Source: CAD feature listing. Evaluate the final solid. Frame: model axes, mm. Give positions to 0.01 mm unless a question says otherwise; leave off trailing zeros. Write each loop counter-clockwise with the first axis right and the second up, starting at its lowest first coordinate (ties: lowest second). Pieces come first, ordered by that corner, then holes. Notation, with made-up numbers: (71, 56) -> (120, 56) arc R28 cw to (120, 84) -> close; hole circle Ø9 at (-9.75, 31.25). An arc over 180 degrees is marked (long way). Answer as a JSON object with one key per item and string values. Group by question number.
Item 1: Section query B-B on x = 134.5. Return the cut outline in (y, z).
Item 2: Section query A-A on x = 260. Return the cut outline in (y, z).
Item 3: Section query C-C on y = 0.95. Give the number of separate pieces and of enclosed holes in the cut face, plus the area to 3 significant figures.
Item 4: First-contact query: pin 1 Ø1.5 at (y, z) = (1, -13) entering from +X; pin 2 Ø1.5 at (x, y) = (202.5, 1.5) entering from -Z; pin 3 Ø1.5 at (y, z) = (2, -16) entering from -X. Flat tips, straight axial feed; report the tip coordinate or a pass-through.
Item 5: Ray query, probe 1 along X at (y, z) = (2.1, -16); probe 2 along X at (y, z) = (2.75, -6.75); probe 3 along Z at (x, y) = (35.5, 1). Return the intervals inside material, ascending. Write a range as from..to.
Item 6: Section query D-D on x = 51. Return the cut outline in (y, z).
from build123d import *

# Parameters (mm, degrees)
SKICA1_W                 = 285
SKICA1_H                 = 15
P_IDAT_VYSUNUT_M1_DEPTH  = 3
SKICA2_W                 = 25
SKICA2_H                 = 3
SKICA2_W_2               = 3
SKICA2_H_2               = 5
P_IDAT_VYSUNUT_M2_DEPTH  = 3
SKICA3_W                 = 25
SKICA3_H                 = 5
ODEBRAT_VYSUNUT_M1_DEPTH = 289.577545904


with BuildPart() as part:
    # Skica1 → Přidat vysunutím1 (new body)
    with BuildSketch(Plane(origin=(0, 0, 0), x_dir=(1, 0, 0), z_dir=(0, 1, 0))):
        with Locations((142.5, 7.5)):
            Rectangle(SKICA1_W, SKICA1_H)
    extrude(amount=P_IDAT_VYSUNUT_M1_DEPTH)

    # Skica2 → Přidat vysunutím2 (add)
    with BuildSketch(Plane(origin=(0, 0, 0), x_dir=(1, 0, 0), z_dir=(0, 1, 0))):
        with Locations((67.5, 16.5)):
            Rectangle(SKICA2_W, SKICA2_H)
        with Locations((-1.5, 7.5)):
            Rectangle(SKICA2_W_2, SKICA2_H_2)
        with Locations((17.5, 16.5)):
            Rectangle(SKICA2_W, SKICA2_H)
        with Locations((117.5, 16.5)):
            Rectangle(SKICA2_W, SKICA2_H)
        with Locations((167.5, 16.5)):
            Rectangle(SKICA2_W, SKICA2_H)
        with Locations((286.5, 7.5)):
            Rectangle(SKICA2_W_2, SKICA2_H_2)
        with Locations((217.5, 16.5)):
            Rectangle(SKICA2_W, SKICA2_H)
        with Locations((267.5, 16.5)):
            Rectangle(SKICA2_W, SKICA2_H)
    extrude(amount=P_IDAT_VYSUNUT_M2_DEPTH)

    # Skica3 → Odebrat vysunutím1 (cut, through all)
    with BuildSketch(Plane(origin=(0, 0, 0), x_dir=(1, 0, 0), z_dir=(0, 1, 0))):
        with Locations((27.5, 7.5)):
            Rectangle(SKICA3_W, SKICA3_H)
        with Locations((85, 7.5)):
            Rectangle(SKICA3_W, SKICA3_H)
        with Locations((142.5, 7.5)):
            Rectangle(SKICA3_W, SKICA3_H)
        with Locations((200, 7.5)):
            Rectangle(SKICA3_W, SKICA3_H)
        with Locations((257.5, 7.5)):
            Rectangle(SKICA3_W, SKICA3_H)
    extrude(amount=ODEBRAT_VYSUNUT_M1_DEPTH, mode=Mode.SUBTRACT)


solid = part.part
Worked answers:
{
 "1": {"outline": "(0, -15) -> (3, -15) -> (3, -10) -> (0, -10) -> close; (0, -5) -> (3, -5) -> (3, 0) -> (0, 0) -> close"},
 "2": {"outline": "(0, -18) -> (3, -18) -> (3, -10) -> (0, -10) -> close; (0, -5) -> (3, -5) -> (3, 0) -> (0, 0) -> close"},
 "3": {"separate pieces": "1", "enclosed holes": "5", "area": "4,130 mm^2"},
 "4": {"pin 1": "x = 285", "pin 2": "z = -15", "pin 3": "x = 5"},
 "5": {"probe 1": "5..30, 55..80, 105..130, 155..180, 205..230, 255..280", "probe 2": "-3..15, 40..72.5, 97.5..130, 155..187.5, 212.5..245, 270..288", "probe 3": "-15..-10, -5..0"},
 "6": {"outline": "(0, -15) -> (3, -15) -> (3, 0) -> (0, 0) -> close"}
}
